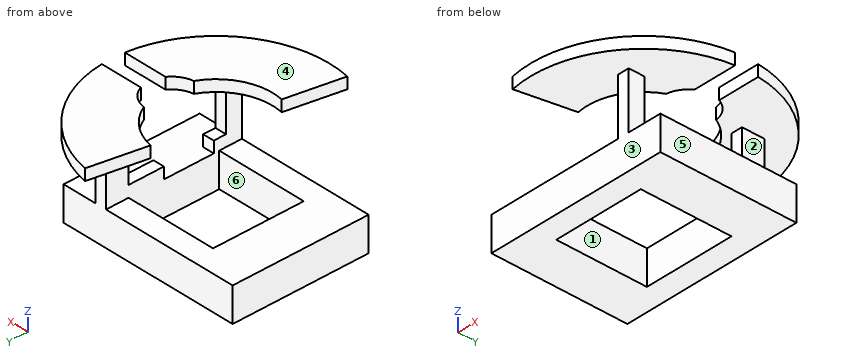
from build123d import *

# Parameters (mm, degrees)
SKETCH2_W           = 60
SKETCH2_H           = 80
SKETCH2_W_2         = 40
SKETCH2_H_2         = 40
BOSS_EXTRUDE1_DEPTH = 15
SKETCH6_W           = 5
SKETCH6_H           = 25.6
SKETCH6_H_2         = 12.4
BOSS_EXTRUDE4_DEPTH = 5
SKETCH8_W           = 5
SKETCH8_H           = 7
BOSS_EXTRUDE5_DEPTH = 20
SKETCH9_W           = 5
SKETCH9_H           = 10
BOSS_EXTRUDE6_DEPTH = 20
BOSS_EXTRUDE7_DEPTH = 5


with BuildPart() as part:
    # Sketch2 → Boss-Extrude1 (new body)
    with BuildSketch(Plane(origin=(0, 0, 0), x_dir=(0, 1, 0), z_dir=(0, 0, 1))):
        Rectangle(SKETCH2_W, SKETCH2_H)
        Rectangle(SKETCH2_W_2, SKETCH2_H_2, mode=Mode.SUBTRACT)
    extrude(amount=BOSS_EXTRUDE1_DEPTH)

    # Sketch6 → Boss-Extrude4 (add)
    with BuildSketch(Plane.XY.offset(15)):
        with Locations((22.5, 17.2)):
            Rectangle(SKETCH6_W, SKETCH6_H)
        with Locations((22.5, -23.8)):
            Rectangle(SKETCH6_W, SKETCH6_H_2)
    extrude(amount=BOSS_EXTRUDE4_DEPTH)

    # Sketch8 → Boss-Extrude5 (add)
    with BuildSketch(Plane.XY.offset(20)):
        with Locations((22.5, -26.5)):
            Rectangle(SKETCH8_W, SKETCH8_H)
    extrude(amount=BOSS_EXTRUDE5_DEPTH)

    # Sketch9 → Boss-Extrude6 (add)
    with BuildSketch(Plane.XY.offset(20)):
        with Locations((22.5, 25)):
            Rectangle(SKETCH9_W, SKETCH9_H)
    extrude(amount=BOSS_EXTRUDE6_DEPTH)

    # Sketch10 → Boss-Extrude7 (add)
    with BuildSketch(Plane.XY.offset(40)):
        with BuildLine():
            Line((-9.424890685, -49.103680469), (-4.712445342, -24.551840234))
            ThreePointArc((-4.712445342, -24.551840234), (11.141961637, -22.379827767), (22.431197476, -11.038178282))
            ThreePointArc((22.431197476, -11.038178282), (26.961461335, -9.399504495), (30.374950987, -6))
            Line((30.374950987, -6), (49.638694584, -6))
            ThreePointArc((49.638694584, -6), (29.474893104, -40.388496834), (-9.424890685, -49.103680469))
        make_face()
        with BuildLine():
            Line((4.712445342, 24.551840234), (9.424890685, 49.103680469))
            ThreePointArc((9.424890685, 49.103680469), (37.23787997, 33.366754342), (49.839743178, 4))
            Line((49.839743178, 4), (31.386996968, 4))
            ThreePointArc((31.386996968, 4), (27.877602661, 8.751473456), (22.431197476, 11.038178282))
            ThreePointArc((22.431197476, 11.038178282), (15.160775086, 19.878402823), (4.712445342, 24.551840234))
        make_face()
    extrude(amount=BOSS_EXTRUDE7_DEPTH)


solid = part.part
The model under review builds one solid part; all positions refer to its coordinate system, in mm. Face numbers are marked on the shaded views. A direction names the side the tool comes from. Round coordinates to 2 decimals unless told otherwise and drop trailing zeros. Loops run counter-clockwise (first coordinate to the right, second up) from the corner with the lowest first, then second, coordinate; pieces in that order, holes last. Notation, with made-up numbers: M -33,24.25 L -8,24.25 A20 ccw -8,38.25 Z; hole C -37,52 d10. An arc over 180 degrees is marked long. Answer as a JSON object with one key per item and string values.
Item 1: We need section A-A, the plane x = -11.5. State the section outline as (y, z) points, and give its area (3 significant figures).
Check sheet entries:
{"outline": "M -30,0 L -20,0 L -20,15 L -30,15 Z; M 20,0 L 30,0 L 30,15 L 20,15 Z", "area": "300 mm2"}
Item 2: The part is to be moulded in two halves that separate along X. For the marked faces 4, 5 and 6, say which applies: +X half, -X half, draft (parallel to the pull), parting line (faces both ways), or undercut.
Check sheet entries:
{"face 4": "draft", "face 5": "+X half", "face 6": "undercut"}
Item 3: We need section D-D, the plane y = 17. State the section outline as (x, z) points, and give its area (3 significant figures).
Check sheet entries:
{"outline": "M -40,0 L -20,0 L -20,15 L -40,15 Z; M 18.33,40 L 47.02,40 L 47.02,45 L 18.33,45 Z; M 20,0 L 40,0 L 40,15 L 25,15 L 25,20 L 20,20 Z", "area": "768 mm2"}
Item 4: Clearance check with flat-ended pins moving along their axes: P1, Ø1.5, axis at x = 21.5, z = 18, coming from the -Y side; P2, Ø5, axis at y = 32.5, z = 39.5, coming from the +X side; P3, Ø22, axis at x = 7.5, y = -25, coming from the -Z side; P4, Ø16.5, axis at y = -3.5, z = 5.5, coming from the +X side. State where each tip first meets the part, or that it passes through.
Check sheet entries:
{"P1": "y = -30", "P2": "x = 39.96", "P3": "z = 0", "P4": "x = 40"}
Item 5: We need section B-B, the plane z = 18. State the section outline as (x, y) points, and give its area (3 significant figures).
Check sheet entries:
{"outline": "M 20,-30 L 25,-30 L 25,-17.6 L 20,-17.6 Z; M 20,4.4 L 25,4.4 L 25,30 L 20,30 Z", "area": "190 mm2"}
Item 6: We need section C-C, the plane x = 16.5. State the section outline as (y, z) points.
Check sheet entries:
{"outline": "M -47.2,40 L -18.78,40 L -18.78,45 L -47.2,45 Z; M -30,0 L -20,0 L -20,15 L -30,15 Z; M 18.78,40 L 47.2,40 L 47.2,45 L 18.78,45 Z; M 20,0 L 30,0 L 30,15 L 20,15 Z"}
Item 7: For line 1 along Y through (x, z) = (23.5, 36.5); line 2 along Z through (x, y) = (32, -9); line 3 along X through (y, z) = (0, 6), list the stretches that pass through material, from the lowest coordinate up.
Check sheet entries:
{"line 1": "-30 to -23, 20 to 30", "line 2": "0 to 15, 40 to 45", "line 3": "-40 to -20, 20 to 40"}
Item 8: Tool access review of the marked faces 1, 2 and 3: name each direction out of +Z, -Z, +X, -X, +Y, -Y from which nothing blocks a thin tool from reaching the whole face with its end or side.
Check sheet entries:
{"face 1": "+Z, -Z", "face 2": "+X, +Y, -Y", "face 3": "-Z, +X, -X, -Y"}
